The model under review builds one solid part; all positions refer to its coordinate system, in mm. A direction names the side the tool comes from. Round coordinates to 2 decimals unless told otherwise and drop trailing zeros. Write each loop counter-clockwise with the first axis right and the second up, starting at its lowest first coordinate (ties: lowest second). Pieces come first, ordered by that corner, then holes. Notation, with made-up numbers: M -23,-39 L 0,-39 A15 cw 0,-27 Z; hole C -13,-5 d6. An arc over 180 degrees is marked long. One line per item, written item: value. Start each with the question number.
1) For P1, Ø3, axis at x = 21, y = 17.5, coming from the -Z side; P2, Ø0.9, axis at x = 18.5, z = 2, coming from the -Y side; P3, Ø11, axis at x = -22.5, y = 6.5, coming from the +Z side; P4, Ø2, axis at x = -15, y = 35, coming from the +Z side, all flat-tipped, find the tip position at first contact; note any pin that passes through.
2) Tool access review of faces 4 (the face through (-15.66, 11.81, 11.38)), 5 (the face through (-33.533, 2.377, 1.479)), 6 (the face through (-26, 8.57, 1.52)), 7 (the face through (-24, 22, 1)): name each direction out of +Z, -Z, +X, -X, +Y, -Y from which nothing blocks a thin tool from reaching the whole face with its end or side.
3) Mouldability with a two-part tool opening along X and no side actions: class faces 1 (the face through (-35, 10, 1)), 2 (the face through (-14, 18, 0)), 3 (the face through (15.07, 38, 9.86)) as +X half, -X half, draft (parallel to the pull), parting line (faces both ways), or undercut.
4) Take a section at A-A, the plane y = 27. Write out the cut boundary in (x, z).
5) Wall thickness on probe 1 along X at (y, z) = (17, 14.25); probe 2 along X at (y, z) = (16.5, 1); probe 3 along Y at (x, z) = (-4, 5.5): over which ranges is each line inside the solid? List them lowest first.
6) Take a section at C-C, the plane x = 33.5. Write out the cut boundary in (y, z).
7) Take a section at D-D, the plane z = 19.25. Write out the cut boundary in (x, y).
8) Take a section at B-B, the plane y = 12. Write out the cut boundary in (x, z), and give its area (3 significant figures).
from build123d import *

# Parameters (mm, degrees)
F2_DEPTH     = 25
F3_DEPTH     = 3
F4_DEPTH     = 25
F5_R         = 4.99999
F6_T1_DEPTH  = 25
F6_T3_DEPTH  = 25
F6_T5_DEPTH  = 50
F6_T7_DEPTH  = 33.4564392374
F6_T9_DEPTH  = 50
F6_T11_DEPTH = 33.4564392374
F7_T1_DEPTH  = 19.917424305
F7_T3_DEPTH  = 23
F7_T6_ANGLE  = 89.9999999974
F7_T8_ANGLE  = 89.9999999974
F7_T10_ANGLE = 209.6926070845
F7_T12_ANGLE = 209.6926070845


# Not quite as in the source:
# - a fillet or chamfer that OpenCascade refuses, or shapes differently, is made with other operations: its cross-section is extruded or revolved along the edge and cut away or added
# - a fillet or chamfer is up to 0.001 mm smaller than in the source, because OpenCascade refuses the exact size


with BuildPart() as f2:
    # F0 (on Top) → F2 (new body)
    with BuildSketch(Plane.XY):
        Polygon((16.5, 39.5), (0, 39.5), (-16.5, 39.5), (-16.5, 22), (-16.5, 10), (-13.5, 10), (-13.5, 36.5), (0, 36.5), (13.5, 36.5), (13.5, 10), (16.5, 10), (16.5, 22), align=None)
    extrude(amount=F2_DEPTH)

    # F0 (on Top) → F3 (join)
    with BuildSketch(Plane.XY):
        Polygon((-16.5, 10), (-16.5, 22), (-37.5, 22), (-37.5, 0), (-27.5, 0), (-27.5, 10), align=None)
        Polygon((37.5, 22), (16.5, 22), (16.5, 10), (27.5, 10), (27.5, 0), (37.5, 0), align=None)
    extrude(amount=F3_DEPTH)

    # F1 (on Top) → F4 (cut)
    with BuildSketch(Plane.XY):
        with BuildLine():
            Line((35, 3.8767794613), (35, 15.8767794613))
            ThreePointArc((35, 15.8767794613), (33.5, 17.3767794613), (32, 15.8767794613))
            Line((32, 15.8767794613), (32, 3.8767794613))
            ThreePointArc((32, 3.8767794613), (33.5, 2.3767794613), (35, 3.8767794613))
        make_face()
        with BuildLine():
            ThreePointArc((-32, 15.8767794613), (-33.5, 17.3767794613), (-35, 15.8767794613))
            Line((-35, 15.8767794613), (-35, 3.8767794613))
            ThreePointArc((-35, 3.8767794613), (-33.5, 2.3767794613), (-32, 3.8767794613))
            Line((-32, 3.8767794613), (-32, 15.8767794613))
        make_face()
    extrude(amount=F4_DEPTH, mode=Mode.SUBTRACT)

    # F5 (radius 5 in the source; OpenCascade refuses exactly that, so slightly less here)
    f5_edges = [f2.edges().sort_by_distance(p)[0] for p in [
        (-37.5, 0, 1.5),
        (-27.5, 0, 1.5),
        (-37.5, 22, 1.5),
        (37.5, 22, 1.5),
        (37.5, 0, 1.5),
        (27.5, 0, 1.5),
        (27.5, 10, 1.5),
        (-27.5, 10, 1.5),
    ]]
    fillet(f5_edges, radius=F5_R)

    # F6: fillet of radius 5 on 6 edges, made by hand

    # F6_s2 → F6_t1 (join)
    with BuildSketch(Plane.XY):
        with BuildLine():
            ThreePointArc((13.5, 31.5), (12.0355339059, 35.0355339059), (8.5, 36.5))
            Line((8.5, 36.5), (13.5, 36.5))
            Line((13.5, 36.5), (13.5, 31.5))
        make_face()
    extrude(amount=F6_T1_DEPTH)

    # F6_s4 → F6_t3 (join)
    with BuildSketch(Plane.XY):
        with BuildLine():
            ThreePointArc((-8.5, 36.5), (-12.0355339059, 35.0355339059), (-13.5, 31.5))
            Line((-13.5, 31.5), (-13.5, 36.5))
            Line((-13.5, 36.5), (-8.5, 36.5))
        make_face()
    extrude(amount=F6_T3_DEPTH)

    # F6_s6 → F6_t5 (cut)
    with BuildSketch(Plane.XY.offset(-12.5)):
        with BuildLine():
            ThreePointArc((16.5, 34.5), (15.0355339059, 38.0355339059), (11.5, 39.5))
            Line((11.5, 39.5), (16.5, 39.5))
            Line((16.5, 39.5), (16.5, 34.5))
        make_face()
    extrude(amount=F6_T5_DEPTH, mode=Mode.SUBTRACT)

    # F6_s8 → F6_t7 (cut)
    with BuildSketch(Plane.XY.offset(3)):
        with BuildLine():
            ThreePointArc((13.5, 10), (15.6833001327, 11.8439629074), (16.5, 14.582575695))
            Line((16.5, 14.582575695), (16.5, 10))
            Line((16.5, 10), (13.5, 10))
        make_face()
    extrude(amount=F6_T7_DEPTH, mode=Mode.SUBTRACT)

    # F6_s10 → F6_t9 (cut)
    with BuildSketch(Plane.XY.offset(-12.5)):
        with BuildLine():
            ThreePointArc((-11.5, 39.5), (-15.0355339059, 38.0355339059), (-16.5, 34.5))
            Line((-16.5, 34.5), (-16.5, 39.5))
            Line((-16.5, 39.5), (-11.5, 39.5))
        make_face()
    extrude(amount=F6_T9_DEPTH, mode=Mode.SUBTRACT)

    # F6_s12 → F6_t11 (cut)
    with BuildSketch(Plane.XY.offset(3)):
        with BuildLine():
            ThreePointArc((-13.5, 10), (-15.6833001327, 11.8439629074), (-16.5, 14.582575695))
            Line((-16.5, 14.582575695), (-16.5, 10))
            Line((-16.5, 10), (-13.5, 10))
        make_face()
    extrude(amount=F6_T11_DEPTH, mode=Mode.SUBTRACT)

    # F7: fillet of radius 5 on 3 edges, made by hand

    # F7_s2 → F7_t1 (cut)
    with BuildSketch(Plane.XZ.offset(-34.5)):
        with BuildLine():
            ThreePointArc((-11.5, 25), (-15.0355339059, 23.5355339059), (-16.5, 20))
            Line((-16.5, 20), (-16.5, 25))
            Line((-16.5, 25), (-11.5, 25))
        make_face()
        with BuildLine():
            ThreePointArc((11.5, 25), (15.0355339059, 23.5355339059), (16.5, 20))
            Line((16.5, 20), (16.5, 25))
            Line((16.5, 25), (11.5, 25))
        make_face()
    extrude(amount=F7_T1_DEPTH, mode=Mode.SUBTRACT)

    # F7_s4 → F7_t3 (cut)
    with BuildSketch(Plane.YZ.offset(-11.5)):
        with BuildLine():
            ThreePointArc((34.5, 25), (38.0355339059, 23.5355339059), (39.5, 20))
            Line((39.5, 20), (39.5, 25))
            Line((39.5, 25), (34.5, 25))
        make_face()
    extrude(amount=F7_T3_DEPTH, mode=Mode.SUBTRACT)

    # F7_s5 → F7_t6 (revolve, cut)
    with BuildSketch(Plane.YZ.offset(11.4999999999)):
        with BuildLine():
            ThreePointArc((34.5, 25), (38.0355339059, 23.5355339059), (39.5, 20))
            Line((39.5, 20), (39.5, 25))
            Line((39.5, 25), (34.5, 25))
        make_face()
    revolve(axis=Axis((11.4999999999, 34.4999999999, 25), (0, 0, -1)), revolution_arc=F7_T6_ANGLE, mode=Mode.SUBTRACT)

    # F7_s7 → F7_t8 (revolve, cut)
    with BuildSketch(Plane.XZ.offset(-34.4999999999)):
        with BuildLine():
            ThreePointArc((-11.5, 25), (-15.0355339059, 23.5355339059), (-16.5, 20))
            Line((-16.5, 20), (-16.5, 25))
            Line((-16.5, 25), (-11.5, 25))
        make_face()
    revolve(axis=Axis((-11.4999999999, 34.4999999999, 25), (0, 0, -1)), revolution_arc=F7_T8_ANGLE, mode=Mode.SUBTRACT)

    # F7_s9 → F7_t10 (revolve, cut)
    with BuildSketch(Plane.XZ.offset(-14.5825756948)):
        with BuildLine():
            ThreePointArc((16.5, 20), (15.0355339059, 23.5355339059), (11.5, 25))
            Line((11.5, 25), (16.5, 25))
            Line((16.5, 25), (16.5, 20))
        make_face()
    revolve(axis=Axis((11.5000000002, 14.5825756948, 25), (0, 0, -1)), revolution_arc=F7_T10_ANGLE, mode=Mode.SUBTRACT)

    # F7_s11 → F7_t12 (revolve, cut)
    with BuildSketch(Plane(origin=(-9.0966946013, 15.9529859327, 0), x_dir=(0, 0, 1), z_dir=(-0.4953465841, 0.8686954366, 0))):
        with BuildLine():
            ThreePointArc((25, -2.7665684632), (23.5355339059, 0.7689654427), (20, 2.2334315368))
            Line((20, 2.2334315368), (25, 2.2334315368))
            Line((25, 2.2334315368), (25, -2.7665684632))
        make_face()
    revolve(axis=Axis((-11.5000000002, 14.5825756948, 25), (0, 0, -1)), revolution_arc=F7_T12_ANGLE, mode=Mode.SUBTRACT)


solid = f2.part
Checked values:
1. P1: stops at z = 0
1. P2: stops at y = 10
1. P3: stops at z = 3
1. P4: stops at z = 24.31
2. face 4: +Z, -X, -Y
2. face 5: +Z, -Z
2. face 6: +Z, -Z, -Y
2. face 7: +Z, -Z, -X, +Y
3. face 1: undercut
3. face 2: draft
3. face 3: +X half
4. outline: M -16.5,0 L -13.5,0 L -13.5,24.58 A5 ccw -16.5,20 Z; M 13.5,0 L 16.5,0 L 16.5,20 A5 ccw 13.5,24.58 Z
5. probe 1: x = -16.5 to -13.5, 13.5 to 16.5
5. probe 2: x = -37.5 to -34.86, -32.14 to -13.5, 13.5 to 32.14, 34.86 to 37.5
5. probe 3: y = 36.5 to 39.5
6. outline: M 0.1,0 L 2.38,0 L 2.38,3 L 0.1,3 Z; M 17.38,0 L 21.9,0 L 21.9,3 L 17.38,3 Z
7. outline: M -16.5,14.58 A5 ccw -13.5,10 L -13.5,31.5 A5 cw -8.5,36.5 L 8.5,36.5 A5 cw 13.5,31.5 L 13.5,10 A5 ccw 16.5,14.58 L 16.5,34.5 A5 ccw 11.5,39.5 L -11.5,39.5 A5 ccw -16.5,34.5 Z
8. outline: M -37.5,0 L -35,0 L -35,3 L -37.5,3 Z; M -32,0 L -13.5,0 L -13.5,23.79 A4.28 ccw -15.78,20 L -15.78,3 L -32,3 Z; M 13.5,0 L 32,0 L 32,3 L 15.78,3 L 15.78,20 A4.28 ccw 13.5,23.79 Z; M 35,0 L 37.5,0 L 37.5,3 L 35,3 Z
8. area: 216 mm2
